from build123d import *

# Parameters (mm, degrees)
SKETCH_W     = 111.252
SKETCH_H     = 44.45
SKETCH_R     = 1.65
PAD_DEPTH    = 1.5875
SKETCH001_R  = 1.65
SKETCH001_W  = 82.042
SKETCH001_H  = 20.066
POCKET_DEPTH = 1.5885


with BuildPart() as part:
    # Sketch → Pad (new body)
    with BuildSketch(Plane.XY):
        with Locations((1, 1)):
            Rectangle(SKETCH_W, SKETCH_H)
        with Locations((-51.326, 19.925)):
            Circle(SKETCH_R, mode=Mode.SUBTRACT)
        with Locations((53.326, -17.925)):
            Circle(SKETCH_R, mode=Mode.SUBTRACT)
        with Locations((53.326, 19.925)):
            Circle(SKETCH_R, mode=Mode.SUBTRACT)
        with Locations((-51.326, -17.925)):
            Circle(SKETCH_R, mode=Mode.SUBTRACT)
    extrude(amount=PAD_DEPTH)

    # Sketch001 → Pocket (cut, through all)
    with BuildSketch(Plane.XY):
        with Locations((-51.326, 19.925)):
            Circle(SKETCH001_R)
        with Locations((1, 1)):
            Rectangle(SKETCH001_W, SKETCH001_H)
    extrude(amount=POCKET_DEPTH, mode=Mode.SUBTRACT)


solid = part.part
Can you work these out from the model? Positions are in its coordinate system, mm. Give positions to 0.01 mm unless a question says otherwise; leave off trailing zeros. Write each loop counter-clockwise with the first axis right and the second up, starting at its lowest first coordinate (ties: lowest second). Pieces come first, ordered by that corner, then holes. Notation, with made-up numbers: M 52.25,10 L 64.25,10 A22 cw 64.25,37 Z; hole C 51,4 d9. An arc over 180 degrees is marked long. Answer in a Markdown table with one row per item. Add a question column.
Item 1: Imagine slicing it at C-C, the plane z = 0.45. Write out the boundary of the cut face in (x, y) (3 decimals), plus the area to 3 significant figures.
Item 2: For pin 1 Ø2 at (x, y) = (53.326, -17.925) entering from -Z, with a flat end and sliding along its axis, tell me the tip position at first contact or that it passes through.
Item 3: We'd pull the mould along X, two halves only. Please class faces 1 (the cylindrical face through (51.678, 19.998, 0.783)), 2 (the flat face through (0.2, 11.2, 1.588)): released by +X, released by -X, zero draft, split by the parting line, or undercut.
Item 4: Imagine slicing it at B-B, the plane y = 8.5. Write out the boundary of the cut face in (x, z), plus the area to 3 significant figures.
Item 5: Imagine slicing it at A-A, the plane x = 36. Write out the boundary of the cut face in (y, z) (1 decimal).
Item 6: Please list where these lines run through material, in increasing order: L1, parallel to X at y = 20, z = 1.35; L2, parallel to Y at x = -6, z = 1 (3 decimals); L3, parallel to X at y = -0.5, z = 0.2.
Evaluation:
| question | item | result |
|---|---|---|
| 1 | outline | M -54.626,-21.225 L 56.626,-21.225 L 56.626,23.225 L -54.626,23.225 Z; hole C -51.326,-17.925 d3.3; hole C -51.326,19.925 d3.3; hole M -40.021,-9.033 L 42.021,-9.033 L 42.021,11.033 L -40.021,11.033 Z; hole C 53.326,-17.925 d3.3; hole C 53.326,19.925 d3.3 |
| 1 | area | 3,260 mm² |
| 2 | pin 1 | passes through |
| 3 | face 1 | undercut |
| 3 | face 2 | zero draft |
| 4 | outline | M -54.63,0 L -40.02,0 L -40.02,1.59 L -54.63,1.59 Z; M 42.02,0 L 56.63,0 L 56.63,1.59 L 42.02,1.59 Z |
| 4 | area | 46.4 mm² |
| 5 | outline | M -21.2,0 L -9,0 L -9,1.6 L -21.2,1.6 Z; M 11,0 L 23.2,0 L 23.2,1.6 L 11,1.6 Z |
| 6 | L1 | x = -54.63 to -52.97, -49.68 to 51.68, 54.97 to 56.63 |
| 6 | L2 | y = -21.225 to -9.033, 11.033 to 23.225 |
| 6 | L3 | x = -54.63 to -40.02, 42.02 to 56.63 |
